Could you check a few things on this model? Use its own coordinates, in mm. Face numbers are marked on the shaded views. A direction names the side the tool comes from. Round coordinates to 2 decimals unless told otherwise and drop trailing zeros. Loops run counter-clockwise (first coordinate to the right, second up) from the corner with the lowest first, then second, coordinate; pieces in that order, holes last. Notation, with made-up numbers: (10, 60) - (51, 60) arc R18 ccw to (51, 66) - close; hole circle Ø5 at (-28, 53.5). An arc over 180 degrees is marked (long way). Answer as CSV lines item,"result". Start each with the question number.
1) Suppose I cut it at A-A, the plane z = 0. Write out the boundary of the cut face in (x, y), then the cut area to 3 significant figures.
2) Suppose I cut it at C-C, the plane x = 0. Write out the boundary of the cut face in (y, z), then the cut area to 3 significant figures.
3) We'd pull the mould along X, two halves only. Please class the marked faces 1, 2 and 3: pulls with the +X half, pulls with the -X half, needs draft (parallel to the pull), parting line crosses it, or undercut.
4) I'm going to push flat-ended pins straight in: pin 1 Ø3 at (x, y) = (16, 37) entering from -Z; pin 2 Ø10 at (x, z) = (4, -6) entering from +Y; pin 3 Ø10 at (x, y) = (17.5, 37) entering from -Z. Where does each tip first touch, or does it pass through?
5) Which directions (+Z, -Z, +X, -X, +Y, -Y) give clear straight access to the entire face, cutting with the end or side of a thin tool? Please do the marked faces 4, 5 and 6.
6) Suppose I cut it at B-B, the plane y = 0. Write out the boundary of the cut face in (x, z).
7) Please list where these lines run through material, in increasing order: line 1 along Y through (x, z) = (0, -4.5); line 2 along Z through (x, y) = (0.5, 42.5); line 3 along X through (y, z) = (-0.5, 7.25).
8) Suppose I cut it at D-D, the plane z = -3.5. Write out the boundary of the cut face in (x, y), then the cut area to 3 significant figures.
```python
from build123d import *

# Parameters (mm, degrees)
SKETCH2_R           = 11.5
BOSS_EXTRUDE1_DEPTH = 12.5
SKETCH4_R           = 14.5
SKETCH4_R_2         = 13
EXTRUDE_THIN1_DEPTH = 30
SKETCH5_W           = 12.460030261
SKETCH5_H           = 20
CUT_EXTRUDE1_DEPTH  = 1.5
SKETCH8_R           = 1.75
BOSS_EXTRUDE2_DEPTH = 3
CHAMFER1_SIZE       = 1


with BuildPart() as part:
    # Sketch2 → Boss-Extrude1 (new, symmetric)
    with BuildSketch(Plane.XY):
        with BuildLine():
            Line((-7.5, 17.5), (7.5, 17.5))
            ThreePointArc((7.5, 17.5), (14.571067812, 14.571067812), (17.5, 7.5))
            Line((17.5, 7.5), (17.5, -7.5))
            ThreePointArc((17.5, -7.5), (14.571067812, -14.571067812), (7.5, -17.5))
            Line((7.5, -17.5), (-7.5, -17.5))
            ThreePointArc((-7.5, -17.5), (-14.571067812, -14.571067812), (-17.5, -7.5))
            Line((-17.5, -7.5), (-17.5, 7.5))
            ThreePointArc((-17.5, 7.5), (-14.571067812, 14.571067812), (-7.5, 17.5))
        make_face()
        Circle(SKETCH2_R, mode=Mode.SUBTRACT)
    extrude(amount=BOSS_EXTRUDE1_DEPTH, both=True)

    # Sketch4 → Extrude-Thin1 (add)
    with BuildSketch(Plane(origin=(0, 17.5, 0), x_dir=(1, 0, 0), z_dir=(0, 1, 0))):
        Circle(SKETCH4_R)
        Circle(SKETCH4_R_2, mode=Mode.SUBTRACT)
    extrude(amount=EXTRUDE_THIN1_DEPTH)

    # Sketch5 → Cut-Extrude1 (cut, symmetric)
    with BuildSketch(Plane.XY):
        with Locations((15.450437523, 37.5)):
            Rectangle(SKETCH5_W, SKETCH5_H)
    extrude(amount=CUT_EXTRUDE1_DEPTH, both=True, mode=Mode.SUBTRACT)

    # Sketch8 → Boss-Extrude2 (add)
    with BuildSketch(Plane(origin=(0, 0, 1.5), x_dir=(-1, 0, 0), z_dir=(0, 0, -1))):
        with BuildLine():
            Line((-12.91317157, 47.5), (-20.91317157, 47.5))
            ThreePointArc((-20.91317157, 47.5), (-22.327385133, 46.914213562), (-22.91317157, 45.5))
            Line((-22.91317157, 45.5), (-22.91317157, 34.5))
            ThreePointArc((-22.91317157, 34.5), (-22.327385133, 33.085786438), (-20.91317157, 32.5))
            Line((-20.91317157, 32.5), (-12.91317157, 32.5))
            Line((-12.91317157, 32.5), (-12.91317157, 47.5))
        make_face()
        with Locations((-18.91317157, 43.5)):
            Circle(SKETCH8_R, mode=Mode.SUBTRACT)
        with Locations((-18.91317157, 36.5)):
            Circle(SKETCH8_R, mode=Mode.SUBTRACT)
    boss_extrude2 = extrude(amount=-BOSS_EXTRUDE2_DEPTH)

    # Mirror1: Boss-Extrude2 across plane
    add(boss_extrude2.mirror(Plane.XY))

    # Chamfer1
    chamfer1_edges = [part.edges().sort_by_distance(p)[0] for p in [
        (-11.5, 0, -12.5),
        (-11.5, 0, 12.5),
    ]]
    chamfer(chamfer1_edges, length=CHAMFER1_SIZE)


solid = part.part
```
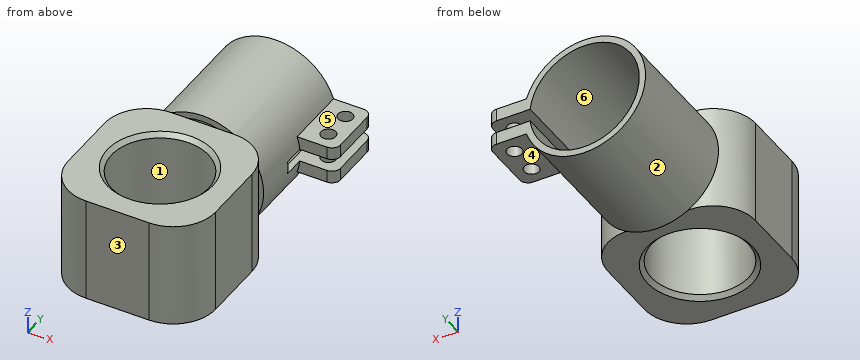
Filled sheet:
1,outline,"(-17.5, -7.5) arc R10 ccw to (-7.5, -17.5) - (7.5, -17.5) arc R10 ccw to (17.5, -7.5) - (17.5, 7.5) arc R10 ccw to (7.5, 17.5) - (-7.5, 17.5) arc R10 ccw to (-17.5, 7.5) - close; (-14.5, 17.5) - (-13, 17.5) - (-13, 47.5) - (-14.5, 47.5) - close; (13, 17.5) - (14.5, 17.5) - (14.5, 27.5) - (13, 27.5) - close; hole circle Ø23 at (0, 0)"
1,area,"784 mm²"
2,outline,"(-17.5, -12.5) - (-12.5, -12.5) - (-11.5, -11.5) - (-11.5, 11.5) - (-12.5, 12.5) - (-17.5, 12.5) - close; (11.5, -11.5) - (12.5, -12.5) - (17.5, -12.5) - (17.5, 12.5) - (12.5, 12.5) - (11.5, 11.5) - close; (17.5, -14.5) - (47.5, -14.5) - (47.5, -13) - (17.5, -13) - close; (17.5, 13) - (47.5, 13) - (47.5, 14.5) - (17.5, 14.5) - close"
2,area,"388 mm²"
3,face 1,"undercut"
3,face 2,"parting line crosses it"
3,face 3,"needs draft"
4,pin 1,"z = -4.5"
4,pin 2,"y = 17.5"
4,pin 3,"z = -7.35"
5,face 4,"-Z, +X, +Y"
5,face 5,"+Z, +X, +Y"
5,face 6,"+Y"
6,outline,"(-17.5, -12.5) - (-12.5, -12.5) - (-11.5, -11.5) - (-11.5, 11.5) - (-12.5, 12.5) - (-17.5, 12.5) - close; (11.5, -11.5) - (12.5, -12.5) - (17.5, -12.5) - (17.5, 12.5) - (12.5, 12.5) - (11.5, 11.5) - close"
7,line 1,"-17.5 to -11.5, 11.5 to 17.5"
7,line 2,"-14.49 to -12.99, 12.99 to 14.49"
7,line 3,"-17.5 to -11.49, 11.49 to 17.5"
8,outline,"(-17.5, -7.5) arc R10 ccw to (-7.5, -17.5) - (7.5, -17.5) arc R10 ccw to (17.5, -7.5) - (17.5, 7.5) arc R10 ccw to (7.5, 17.5) - (-7.5, 17.5) arc R10 ccw to (-17.5, 7.5) - close; (-14.07, 17.5) - (-12.52, 17.5) - (-12.52, 47.5) - (-14.07, 47.5) - close; (12.52, 17.5) - (14.07, 17.5) - (14.07, 32.5) - (20.91, 32.5) arc R2 ccw to (22.91, 34.5) - (22.91, 45.5) arc R2 ccw to (20.91, 47.5) - (12.52, 47.5) - close; hole circle Ø23 at (0, 0); hole circle Ø3.5 at (18.91, 36.5); hole circle Ø3.5 at (18.91, 43.5)"
8,area,"928 mm²"
